from build123d import *

# Parameters (mm, degrees)
SKETCH1_R          = 6.35
EXTRUDE1_DEPTH     = 1.5748
SKETCH2_R          = 14.9225
EXTRUDE2_DEPTH     = 73.914
SKETCH3_R          = 2.3749
EXTRUDE3_DEPTH     = 19.05
CIRPATTERN1_COUNT  = 3
SKETCH14_W         = 3.33891671
SKETCH14_H         = 0.6858
CUT_EXTRUDE3_DEPTH = 7.874
CHAMFER1_SIZE      = 0.254


with BuildPart() as part:
    # Sketch1 → Extrude1 (new body)
    with BuildSketch(Plane.XY):
        with Locations((0, 6.6548)):
            Circle(SKETCH1_R)
    extrude(amount=EXTRUDE1_DEPTH)

    # Sketch2 → Extrude2 (add)
    with BuildSketch(Plane(origin=(0, 0, 0), x_dir=(-1, 0, 0), z_dir=(0, 0, -1))):
        with Locations(Location((0, 0, 0), (0, 0, 180))):
            Circle(SKETCH2_R)
    extrude(amount=EXTRUDE2_DEPTH)

    # Sketch3 → Extrude3 (add)
    with BuildSketch(Plane.XY):
        with Locations(Location((0, 6.6548, 0), (0, 0, 180))):
            Circle(SKETCH3_R)
    extrude(amount=EXTRUDE3_DEPTH)

    # Sketch9 → Revolve1 (revolve)
    with BuildSketch(Plane(origin=(0, 0, 0), x_dir=(0, 0, -1), z_dir=(1, 0, 0)), mode=Mode.PRIVATE) as revolve1_sk:
        Polygon((73.914, 0), (73.914, 6.35), (75.4888, 6.35), (75.4888, 1.9812), (76.7588, 1.9812), (76.7588, 0), align=None)
    revolve(revolve1_sk.sketch.rotate(Axis((0, 0, -51.186992867), (0, 0, -1)), 90), axis=Axis((0, 0, -51.186992867), (0, 0, -1)))

    # Sketch13 → Revolve3 (revolve)
    with BuildSketch(Plane(origin=(0, 0, 0), x_dir=(0, 0, -1), z_dir=(1, 0, 0)), mode=Mode.PRIVATE) as revolve3_sk:
        Polygon((0, 14.9225), (0, 17.399), (22.509169763, 17.399), (24.5872, 14.9225), align=None)
    revolve(revolve3_sk.sketch.rotate(Axis((0, 0, 4.819894785), (0, 0, -1)), 90), axis=Axis((0, 0, 4.819894785), (0, 0, -1)))

    # Sketch7 → Cut-Revolve1 (revolve, cut)
    with BuildSketch(Plane(origin=(0, 0, 0), x_dir=(0, 0, -1), z_dir=(-0.9659258262890681, -0.2588190451025213, 0)), mode=Mode.PRIVATE) as cut_revolve1_sk:
        Polygon((-0.381, 13.4874), (5.334, 13.4874), (5.334, 14.566096168), (5.17525, 14.566096168), (4.9768125, 14.9098), (4.8974375, 14.9098), (4.699, 14.566096168), (4.54025, 14.566096168), (4.3418125, 14.9098), (4.2624375, 14.9098), (4.064, 14.566096168), (3.90525, 14.566096168), (3.7068125, 14.9098), (3.6274375, 14.9098), (3.429, 14.566096168), (3.27025, 14.566096168), (3.0718125, 14.9098), (2.9924375, 14.9098), (2.794, 14.566096168), (2.63525, 14.566096168), (2.4368125, 14.9098), (2.3574375, 14.9098), (2.159, 14.566096168), (2.00025, 14.566096168), (1.8018125, 14.9098), (1.7224375, 14.9098), (1.524, 14.566096168), (1.36525, 14.566096168), (1.1668125, 14.9098), (1.0874375, 14.9098), (0.889, 14.566096168), (0.73025, 14.566096168), (0.5318125, 14.9098), (0.4524375, 14.9098), (0.254, 14.566096168), (0.09525, 14.566096168), (-0.1031875, 14.9098), (-0.1825625, 14.9098), (-0.381, 14.566096168), align=None)
    cut_revolve1 = revolve(cut_revolve1_sk.sketch.rotate(Axis((3.490795989, -13.027827989, 0.218691166), (0, 0, -1)), 285), axis=Axis((3.490795989, -13.027827989, 0.218691166), (0, 0, -1)), mode=Mode.SUBTRACT)

    # CirPattern1: Cut-Revolve1 ×3 about axis
    cirpattern1_axis = Axis((0, 0, 0), (0, 0, 1))
    for i in range(1, CIRPATTERN1_COUNT):
        add(cut_revolve1.rotate(cirpattern1_axis, i * 360 / CIRPATTERN1_COUNT), mode=Mode.SUBTRACT)

    # Sketch14 → Cut-Extrude3 (cut)
    with BuildSketch(Plane.XY.offset(19.05)):
        with Locations((0, 8.6868)):
            Rectangle(SKETCH14_W, SKETCH14_H)
    extrude(amount=-CUT_EXTRUDE3_DEPTH, mode=Mode.SUBTRACT)

    # Chamfer1
    chamfer1_edges = [part.edges().sort_by_distance(p)[0] for p in [
        (0.915246787, 4.463345385, 19.05),
        (-1.9812, 0, -76.7588),
    ]]
    chamfer(chamfer1_edges, length=CHAMFER1_SIZE)


solid = part.part
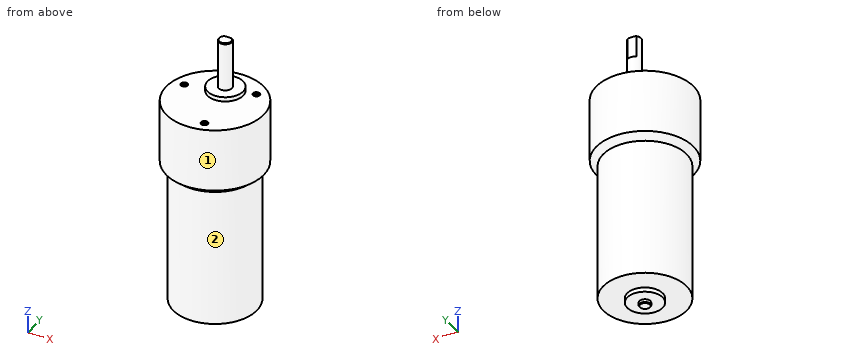
The listing builds one solid part. Answer for the finished solid, in the listing's coordinates (mm). Face numbers are marked on the shaded views. A direction names the side the tool comes from. Coordinates: 2 decimals unless noted, no trailing zeros. Order: outer loops, then holes, each group sorted by start corner. A loop starts at its lowest first (then second) coordinate and runs counter-clockwise, first axis right, second up.
Q1. Consider line 1 (Z direction, x = 7.5, y = -3); line 2 (Z direction, x = -3.5, y = 11.5); line 3 (Y direction, x = 0.5, z = -12.5). Determine where each line is inside the solid, lowest interval first.
Q2. Which of the six approach directions +Z, -Z, +X, -X, +Y, -Y give full straight-line access (tool end or side, diameter ignored) to the marked faces 1 and 2?
Q3. Given P1, Ø5, axis at x = -12.5, z = -14.5, coming from the -Y side; P2, Ø3.5, axis at x = -13.03, y = 3.49, coming from the +Z side; P3, Ø2.5, axis at x = 3.49, y = -13.03, coming from the -Z side, each flat-ended and moving along its own axis, determine where each tip first touches the part or whether it passes through.
Q4. A cutting plane is placed at B-B, the plane z = -18.5. Write down the section's boundary in (x, y).
Q5. A cutting plane is placed at C-C, the plane z = -65.5. Write down the section's boundary in (x, y) (1 decimal).
Answers follow:
1. line 1: z = -73.91 to 0
1. line 2: z = -73.91 to 1.57
1. line 3: y = -17.39 to 17.39
2. face 1: +Z, -Z
2. face 2: -Z
3. P1: stops at y = -14.24
3. P2: stops at z = 0
3. P3: stops at z = -73.91
4. outline: circle Ø34.8 at (0, 0)
5. outline: circle Ø29.8 at (0, 0)
